from build123d import *

# Parameters (mm, degrees)
ESBO_O1_W             = 20
ESBO_O1_H             = 70
FLANGE_BASE1_DEPTH    = 20
ESBO_O2_R             = 4.775
CORTE_EXTRUS_O1_DEPTH = 5.75
ESBO_O3_R             = 2.65
CORTE_EXTRUS_O2_DEPTH = 40.090440008
ESBO_O4_R             = 4
CORTE_EXTRUS_O3_DEPTH = 46
ESBO_O6_R             = 1.65
CORTE_EXTRUS_O4_DEPTH = 10
ESBO_O8_R             = 4.25
CORTE_EXTRUS_O6_DEPTH = 5


# Sheet-metal steps are written as plain solids
with BuildPart() as part:
    # Esboço1 → Flange-base1 (new body)
    with BuildSketch(Plane(origin=(0, 0, 0), x_dir=(1, 0, 0), z_dir=(0, 1, 0))):
        Rectangle(ESBO_O1_W, ESBO_O1_H)
    extrude(amount=-FLANGE_BASE1_DEPTH)

    # Esboço2 → Corte-extrusão1 (cut)
    with BuildSketch(Plane(origin=(0, 0, 0), x_dir=(1, 0, 0), z_dir=(0, 1, 0))):
        with Locations(Location((0, 13, 0), (0, 0, 270))):
            Circle(ESBO_O2_R)
        with Locations(Location((0, -13, 0), (0, 0, 270))):
            Circle(ESBO_O2_R)
    extrude(amount=-CORTE_EXTRUS_O1_DEPTH, mode=Mode.SUBTRACT)

    # Esboço3 → Corte-extrusão2 (cut, through all)
    with BuildSketch(Plane(origin=(0, -5.75, 0), x_dir=(1, 0, 0), z_dir=(0, 1, 0))):
        with Locations(Location((0, 13, 0), (0, 0, 270))):
            Circle(ESBO_O3_R)
        with Locations(Location((0, -13, 0), (0, 0, 270))):
            Circle(ESBO_O3_R)
    extrude(amount=-CORTE_EXTRUS_O2_DEPTH, mode=Mode.SUBTRACT)

    # Esboço4 → Corte-extrusão3 (cut, through all)
    with BuildSketch(Plane.ZY.offset(10)):
        with Locations((26, -10)):
            Circle(ESBO_O4_R)
        with Locations((-26, -10)):
            Circle(ESBO_O4_R)
    extrude(amount=-CORTE_EXTRUS_O3_DEPTH, mode=Mode.SUBTRACT)

    # Esboço6 → Corte-extrusão4 (cut)
    with BuildSketch(Plane(origin=(0, 0, 0), x_dir=(1, 0, 0), z_dir=(0, 1, 0))):
        with Locations(Location((0, -26, 0), (0, 0, 270))):
            Circle(ESBO_O6_R)
        with Locations(Location((0, 26, 0), (0, 0, 270))):
            Circle(ESBO_O6_R)
    extrude(amount=-CORTE_EXTRUS_O4_DEPTH, mode=Mode.SUBTRACT)

    # Esboço8 → Corte-extrusão6 (cut)
    with BuildSketch(Plane(origin=(10, 0, 0), x_dir=(0, 0, -1), z_dir=(1, 0, 0))):
        with Locations((0, -10)):
            Circle(ESBO_O8_R)
    extrude(amount=-CORTE_EXTRUS_O6_DEPTH, mode=Mode.SUBTRACT)


solid = part.part
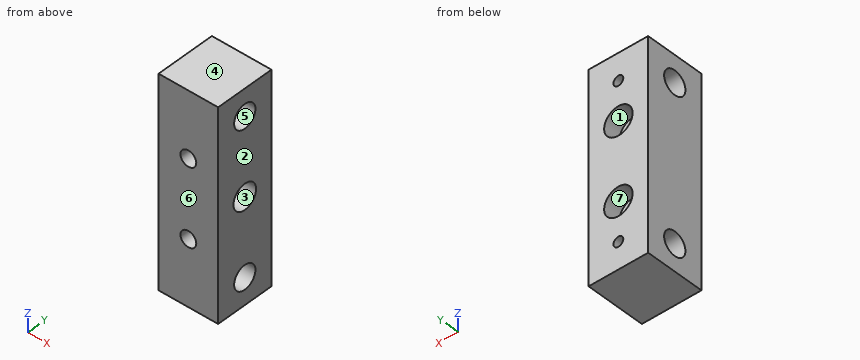
Geometry: final body of the model. Coordinates: model frame, mm. Face numbers are marked on the shaded views. A direction names the side the tool comes from. Coordinates: 2 decimals unless noted, no trailing zeros. Loops run counter-clockwise (first coordinate to the right, second up) from the corner with the lowest first, then second, coordinate; pieces in that order, holes last. Notation, with made-up numbers: M -18.5,59.25 L 2.5,59.25 A36 ccw 2.5,96.25 Z; hole C 71,-35.5 d3. An arc over 180 degrees is marked long. One line per item, written item: value. Start each with the question number.
1) Cut plane C-C (x = 0). Return loops of the section in (y, z) (3 decimals).
2) Cut plane A-A (y = -10). Return loops of the section in (x, z), then the cut area to 3 significant figures.
3) Reachability of the marked faces 1, 2 and 3 from +Z, -Z, +X, -X, +Y, -Y: full face, straight path, thin tool, end or side. Return the list, or none.
4) Material intervals for L1, parallel to X at y = -1.75, z = -13 (3 decimals); L2, parallel to X at y = -12.75, z = -13; L3, parallel to Z at x = -3, y = -3.5, sorted ascending. Write a range as from..to.
5) Pin query (flat end, axial travel): P1, Ø7, axis at x = 0, z = -13, coming from the +Y side; P2, Ø3, axis at x = 0, z = -26, coming from the +Y side. Return the tip coordinate at first contact, or that it passes through.
6) Draft query along Z for the marked faces 4, 5, 6 and 7. Return one class per face: released by +Z, released by -Z, zero draft, split by the parting line, or undercut.
7) Cut plane D-D (z = 26). Return loops of the section in (x, y), then the cut area to 3 significant figures.
8) Cut plane B-B (z = 13). Return loops of the section in (x, y) (3 decimals).
Evaluation:
1. outline: M -20,-35 L 0,-35 L 0,-27.65 L -6.356,-27.65 A4 cw long -6.356,-24.35 L 0,-24.35 L 0,-17.775 L -5.75,-17.775 L -5.75,-15.65 L -20,-15.65 Z; M -20,-10.35 L -5.75,-10.35 L -5.75,-8.225 L 0,-8.225 L 0,8.225 L -5.75,8.225 L -5.75,10.35 L -20,10.35 Z; M -20,15.65 L -5.75,15.65 L -5.75,17.775 L 0,17.775 L 0,24.35 L -6.356,24.35 A4 cw long -6.356,27.65 L 0,27.65 L 0,35 L -20,35 Z
2. outline: M -10,-35 L 10,-35 L 10,-30 L -10,-30 Z; M -10,-22 L 10,-22 L 10,-4.25 L 5,-4.25 L 5,4.25 L 10,4.25 L 10,22 L -10,22 Z; M -10,30 L 10,30 L 10,35 L -10,35 Z; hole C 0,-13 d5.3; hole C 0,13 d5.3
2. area: 993 mm^2
3. face 1: +Y
3. face 2: +Z, -Z, +X, +Y, -Y
3. face 3: +X
4. L1: -10..-4.775, 4.775..10
4. L2: -10..-2.65, 2.65..10
4. L3: -35..-16.71, -9.29..9.29, 16.71..35
5. P1: y = -5.75
5. P2: y = -13.71
6. face 4: released by +Z
6. face 5: undercut
6. face 6: zero draft
6. face 7: undercut
7. outline: M -10,-20 L 10,-20 L 10,-14 L -10,-14 Z; M -10,-6 L -1.65,-6 L -1.65,0 L -10,0 Z; M 1.65,-6 L 10,-6 L 10,0 L 1.65,0 Z
7. area: 220 mm^2
8. outline: M -10,-20 L -2.65,-20 L -2.65,-5.75 L -4.775,-5.75 L -4.775,0 L -10,0 Z; M 2.65,-20 L 10,-20 L 10,0 L 4.775,0 L 4.775,-5.75 L 2.65,-5.75 Z
